Answer from the drawing. Dimensions are ordinates in mm from the lowest x, y and z of the part. A direction names the side the tool comes from. Round coordinates to 2 decimals unless told otherwise and drop trailing zeros. Loops run counter-clockwise (first coordinate to the right, second up) from the corner with the lowest first, then second, coordinate; pieces in that order, holes last. Notation, with made-up numbers: M 69.25,-16.5 L 108.25,-16.5 A18 cw 108.25,12.5 Z; hole C 8,19 d5. An arc over 180 degrees is marked long. Answer as CSV lines item,"result".
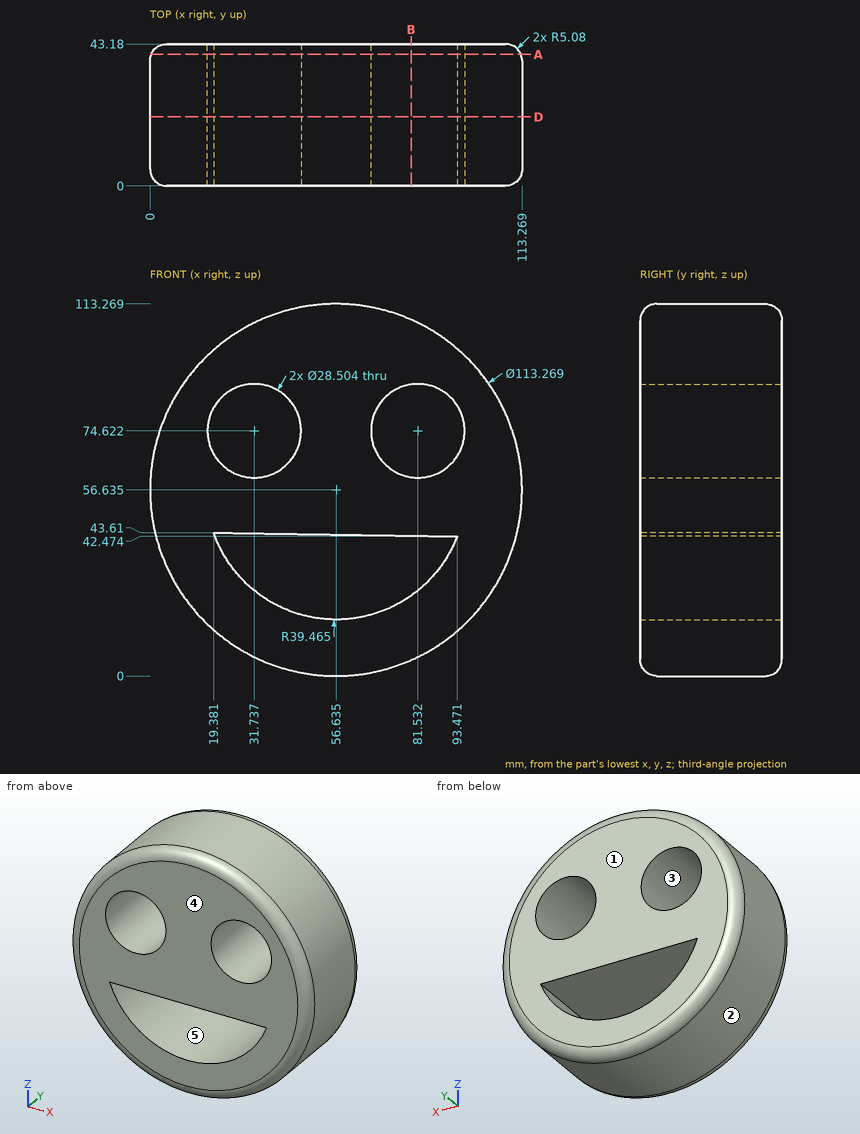
1) Find section D-D, the plane y = 21. Give the vertices of the cut face in (x, z) (1 decimal).
Evaluation:
outline,"C 56.6,56.6 d113.3; hole C 31.7,74.6 d28.5; hole M 19.4,43.6 A39.5 ccw 93.5,42.5 Z; hole C 81.5,74.6 d28.5"
2) Each of these flat-tipped pins is pushed along its axis until it touches: P1, Ø1, axis at y = 9.5, z = 90.5, coming from the -X side; P2, Ø8, axis at x = 53, y = 10, coming from the +Z side; P3, Ø5, axis at y = 8, z = 93, coming from the -X side. Where does it stop, or does it pass through?
Evaluation:
P1,"stops at x = 10.87"
P2,"stops at z = 113.27"
P3,"stops at x = 11.24"
3) Determine the mould class of the marked faces 1, 2 and 3 for opening direction Z: released by +Z, released by -Z, zero draft, split by the parting line, or undercut.
Evaluation:
face 1,"zero draft"
face 2,"split by the parting line"
face 3,"undercut"
4) Find section B-B, the plane x = 79.5. Count the separate pieces of the cut face and the enclosed holes in it.
Evaluation:
separate pieces,"3"
enclosed holes,"0"
5) A tool of negligible diameter and unlimited length cuts with its end or side. For the marked faces 4 and 5, from which of +Z, -Z, +X, -X, +Y, -Y can it reach the whole face along a straight path? Write none if from no direction.
Evaluation:
face 4,"+Z, -Z, +X, -X, -Y"
face 5,"+Y, -Y"
6) Straight lines are drawn through the part: line 1 (Z direction, x = 92.5, y = 36) (1 decimal); line 2 (Z direction, x = 88, y = 13) (1 decimal); line 3 (X direction, y = 20, z = 31) (1 decimal). For each, find the intervals that lie inside material, in ascending order.
Evaluation:
line 1,"z = 12.8 to 40.2, 42.5 to 65.5, 83.7 to 100.5"
line 2,"z = 9.5 to 32.7, 42.6 to 61.9, 87.3 to 103.8"
line 3,"x = 6.1 to 26.6, 86.6 to 107.1"
7) Find section A-A, the plane y = 40. Give the vertices of the cut face in (x, z) (1 decimal).
Evaluation:
outline,"C 56.6,56.6 d112.5; hole C 31.7,74.6 d28.5; hole M 19.4,43.6 A39.5 ccw 93.5,42.5 Z; hole C 81.5,74.6 d28.5"
